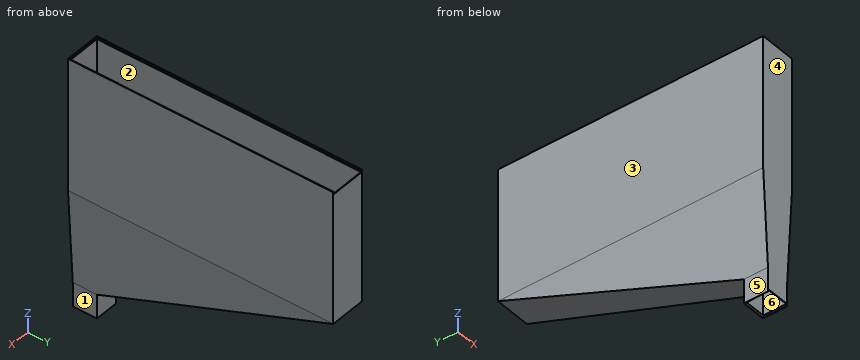
from build123d import *

# Parameters (mm, degrees)
F0_W        = 100
F0_H        = 100
F0_W_2      = 150
F0_H_2      = 550
F1_DEPTH    = 550
F3_DEPTH    = 150
F4_T        = 2.5
F4_T3_DEPTH = 105
F4_T5_DEPTH = 105
F6_DEPTH    = 98.5
F7_W        = 145
F7_H        = 5
F8_DEPTH    = 2.5
F9_DEPTH    = 1099


# Not quite as in the source:
# - a shell that OpenCascade refuses in one call is made with other operations: the cavity is built on its own and cut out


with BuildPart() as f1:
    # F0 (on Front) → F1 (new body, symmetric)
    with BuildSketch(Plane.XZ):
        with Locations((0, -450)):
            Rectangle(F0_W, F0_H)
        with Locations((0, 275)):
            Rectangle(F0_W_2, F0_H_2)
        Polygon((75, 0), (-75, 0), (-50, -400), (50, -400), align=None)
    extrude(amount=F1_DEPTH, both=True)

    # F2 (on face) → F3 (cut)
    with BuildSketch(Plane.YZ.offset(75)):
        Polygon((550, -500), (550, 0), (-450, -400), (-450, -500), align=None)
    extrude(amount=-F3_DEPTH, mode=Mode.SUBTRACT)

    # F4: shell of thickness 2.5, made by hand


with BuildPart() as f4_core1:
    # F4_t2: copy of F1
    add(f1.part)

    # the walls: a layer under each face that stays
    f4_faces = [f4_core1.faces().sort_by_distance(p)[0] for p in [
        (-50, -500, -450),
        (-62.5, 0, -200),
        (0, -550, 25),
        (0, -450, -450),
        (-75, 0, 275),
        (0, 50, -200),
        (50, -500, -450),
        (62.5, 0, -200),
        (75, 0, 275),
        (0, 550, 275),
    ]]
    thicken(f4_faces, amount=-F4_T, mode=Mode.SUBTRACT)

    # F4_s4 → F4_t3 (cut)
    with BuildSketch(Plane.XZ.offset(447.5)):
        Polygon((-50.0499513145, -400.0015594572), (-47.5, -400), (-47.5, -399.9219511453), (-47.5048685538, -399.8440542846), align=None)
        Polygon((50.0499513145, -400.0015594572), (47.5, -400), (47.5, -399.9219511453), (47.5048685538, -399.8440542846), align=None)
    extrude(amount=F4_T3_DEPTH, mode=Mode.SUBTRACT)

    # F4_s6 → F4_t5 (cut)
    with BuildSketch(Plane.YZ.offset(-52.5)):
        Polygon((-449.9657152331, -400.0232119173), (-452.5, -400), (-452.5, -398.3074175964), (-450.9284766909, -397.6788082728), align=None)
    extrude(amount=F4_T5_DEPTH, mode=Mode.SUBTRACT)


with BuildPart() as f1_1:
    add(f1.part)

    # what is left inside the walls is the cavity
    f4_cavity = [f4_core1.part.solids().sort_by_distance(p)[0] for p in [
        (-72.475, 182.5, 275.039024),
    ]]
    add(f4_cavity, mode=Mode.SUBTRACT)

    # F5 (on face) → F6 (cut)
    with BuildSketch(Plane.XZ.offset(550)):
        Polygon((-48.5, -495), (-48.5, -500), (48.5, -500), (48.5, -495), (49.5, -495), (49.5, -490), (-49.5, -490), (-49.5, -495), align=None)
    extrude(amount=-F6_DEPTH, mode=Mode.SUBTRACT)

    # F7 (on face) → F8 (cut)
    with BuildSketch(Plane(origin=(0, 550, 0), x_dir=(-1, 0, 0), z_dir=(0, 1, 0))):
        with Locations((0, 547.5)):
            Rectangle(F7_W, F7_H)
    extrude(amount=-F8_DEPTH, mode=Mode.SUBTRACT)

    # F7 (on face) → F9 (cut)
    with BuildSketch(Plane(origin=(0, 550, 0), x_dir=(-1, 0, 0), z_dir=(0, 1, 0))):
        Polygon((-74, 545), (-74, 540), (74, 540), (74, 545), (72.5, 545), (-72.5, 545), align=None)
    extrude(amount=-F9_DEPTH, mode=Mode.SUBTRACT)


solid = f1_1.part
Input: part model. Units: mm. Frame: model coordinates. Face numbers are marked on the shaded views. A direction names the side the tool comes from. Give positions to 0.01 mm unless a question says otherwise; leave off trailing zeros. Write each loop counter-clockwise with the first axis right and the second up, starting at its lowest first coordinate (ties: lowest second). Pieces come first, ordered by that corner, then holes. Notation, with made-up numbers: (66.25, 37) -> (85.25, 37) arc R11 cw to (85.25, 48) -> close; hole circle Ø10 at (-10.75, 7.25). An arc over 180 degrees is marked (long way). Use one line per item in the form item = value. Start each with the question number.
1) Pin query (flat end, axial travel): pin 1 (2.5 mm diameter, centred on y = -512, z = -492.5, fed in from +X); pin 2 (10 mm diameter, centred on x = -52.5, y = 285, fed in from -Z); pin 3 (3 mm diameter, centred on x = 46, y = 263, fed in from -Z). Return the tip coordinate at first contact, or that it passes through.
2) Section query A-A on x = 11. Return the cut outline in (y, z).
3) Set-up query: the marked faces 1, 2 and 3. Return all of +Z, -Z, +X, -X, +Y, -Y with unobstructed straight access to the full face (end or side cutting, diameter ignored); none if empty.
4) Ray query, probe 1 along X at (y, z) = (118, 478); probe 2 along Y at (x, z) = (-42, 6.5); probe 3 along Y at (x, z) = (0.5, -453). Return the intervals inside material, ascending. Write a range as from..to.
5) Section query D-D on z = -172. Return the cut outline in (x, y).
6) Section query C-C on y = -277. Return the cut outline in (x, z) (3 decimals).
7) Section query B-B on z = 137. Return the cut outline in (x, y), then the cut area to 4 significant figures.
8) Draft query along Y for the marked faces 4, 5 and 6. Return one class per face: pulls with the +Y half, pulls with the -Y half, needs draft (parallel to the pull), parting line crosses it, or undercut.
Outcome:
q1.pin_1 = 50
q1.pin_2 = -108
q1.pin_3 = -115.4
q2.outline = (-550, -490) -> (-547.5, -490) -> (-547.5, 540) -> (-549, 540) -> (-549, 545) -> (-547.5, 545) -> (-547.5, 550) -> (-550, 550) -> close; (-452.5, -490) -> (-451.5, -490) -> (-451.5, -500) -> (-450, -500) -> (-450, -400) -> (550, 0) -> (550, 540) -> (547.5, 540) -> (547.5, 1.69) -> (-452.5, -398.31) -> close
q3.face_1 = -Z, +X, +Y, -Y
q3.face_2 = +Z
q3.face_3 = +Z, -Z, -X, +Y, -Y
q4.probe_1 = -75..-72.5, 72.5..75
q4.probe_2 = -550..-547.5, 547.5..550
q4.probe_3 = -550..-547.5, -452.5..-450
q5.outline = (-64.25, -550) -> (64.25, -550) -> (64.25, 120) -> (-64.25, 120) -> close; hole (-61.75, -547.5) -> (61.75, -547.5) -> (61.75, 113.27) -> (-61.75, 113.27) -> close
q6.outline = (-75, 0) -> (-54.325, -330.8) -> (54.325, -330.8) -> (75, 0) -> (75, 550) -> (72.5, 550) -> (72.5, 545) -> (74, 545) -> (74, 540) -> (72.5, 540) -> (72.5, 0.078) -> (51.988, -328.107) -> (-51.988, -328.107) -> (-72.5, 0.078) -> (-72.5, 540) -> (-74, 540) -> (-74, 545) -> (-72.5, 545) -> (-72.5, 550) -> (-75, 550) -> close
q7.outline = (-75, -550) -> (75, -550) -> (75, 550) -> (-75, 550) -> close; hole (-72.5, -547.5) -> (72.5, -547.5) -> (72.5, 547.5) -> (-72.5, 547.5) -> close
q7.area = 6,225 mm^2
q8.face_4 = pulls with the -Y half
q8.face_5 = needs draft
q8.face_6 = undercut
